Model file for the job. Use its own axes, mm. Face numbers are marked on the shaded views. Coordinates: 2 decimals unless noted, no trailing zeros.
from build123d import *

# Parameters (mm, degrees)
SKETCH_2_R          = 45
CUT_EXTRUDE_1_DEPTH = 15
CUT_EXTRUDE_2_DEPTH = 27
SKETCH_4_W          = 1.65
SKETCH_4_H          = 14.7


with BuildPart() as part:
    # Sketch 1 → Revolve 1 (revolve)
    with BuildSketch(Plane(origin=(0, 0, 0), x_dir=(0, 0, -1), z_dir=(1, 0, 0)), mode=Mode.PRIVATE) as revolve_1_sk:
        Polygon((-15, 19.5), (-15, 6.3), (-14.7, 6), (-0.3, 6), (0, 6.3), (0, 19.5), (-0.803847577, 22.5), (-14.196152423, 22.5), align=None)
    revolve(revolve_1_sk.sketch.rotate(Axis((0, 0, 0), (0, 0, 1)), 270), axis=Axis((0, 0, 0), (0, 0, 1)))

    # Sketch 2 → Cut-Extrude 1 (cut)
    with BuildSketch(Plane.XY):
        Circle(SKETCH_2_R)
        Polygon((-22.5, 0), (-19.377388093, -2.183307284), (-21.935878024, -5.006721014), (-18.405724941, -6.440441708), (-20.271799528, -9.76238413), (-16.511121885, -10.374625492), (-17.591208356, -14.028520542), (-13.788582233, -13.788582233), (-14.028520542, -17.591208356), (-10.374625492, -16.511121885), (-9.76238413, -20.271799528), (-6.440441708, -18.405724941), (-5.006721014, -21.935878024), (-2.183307284, -19.377388093), (0, -22.5), (2.183307284, -19.377388093), (5.006721014, -21.935878024), (6.440441708, -18.405724941), (9.76238413, -20.271799528), (10.374625492, -16.511121885), (14.028520542, -17.591208356), (13.788582233, -13.788582233), (17.591208356, -14.028520542), (16.511121885, -10.374625492), (20.271799528, -9.76238413), (18.405724941, -6.440441708), (21.935878024, -5.006721014), (19.377388093, -2.183307284), (22.5, 0), (19.377388093, 2.183307284), (21.935878024, 5.006721014), (18.405724941, 6.440441708), (20.271799528, 9.76238413), (16.511121885, 10.374625492), (17.591208356, 14.028520542), (13.788582233, 13.788582233), (14.028520542, 17.591208356), (10.374625492, 16.511121885), (9.76238413, 20.271799528), (6.440441708, 18.405724941), (5.006721014, 21.935878024), (2.183307284, 19.377388093), (0, 22.5), (-2.183307284, 19.377388093), (-5.006721014, 21.935878024), (-6.440441708, 18.405724941), (-9.76238413, 20.271799528), (-10.374625492, 16.511121885), (-14.028520542, 17.591208356), (-13.788582233, 13.788582233), (-17.591208356, 14.028520542), (-16.511121885, 10.374625492), (-20.271799528, 9.76238413), (-18.405724941, 6.440441708), (-21.935878024, 5.006721014), (-19.377388093, 2.183307284), align=None, mode=Mode.SUBTRACT)
    extrude(amount=CUT_EXTRUDE_1_DEPTH, mode=Mode.SUBTRACT)

    # Sketch 3 → Cut-Extrude 2 (cut)
    with BuildSketch(Plane.XY):
        with BuildLine():
            Line((-2, 0), (2, 0))
            Line((2, 0), (2, 7.6))
            ThreePointArc((2, 7.6), (1.941421356, 7.741421356), (1.8, 7.8))
            Line((1.8, 7.8), (-1.8, 7.8))
            ThreePointArc((-1.8, 7.8), (-1.941421356, 7.741421356), (-2, 7.6))
            Line((-2, 7.6), (-2, 0))
        make_face()
    extrude(amount=CUT_EXTRUDE_2_DEPTH, mode=Mode.SUBTRACT)

    # Sketch 4 → Hole Wizard M4 _1 (revolve, cut)
    with BuildSketch(Plane(origin=(0, 7.8, 7.5), x_dir=(0, 0, -1), z_dir=(1, 0, 0))):
        with Locations((0.825, 7.35)):
            Rectangle(SKETCH_4_W, SKETCH_4_H)
    revolve(axis=Axis((0, 1.45, 7.5), (0, 1, 0)), mode=Mode.SUBTRACT)


solid = part.part
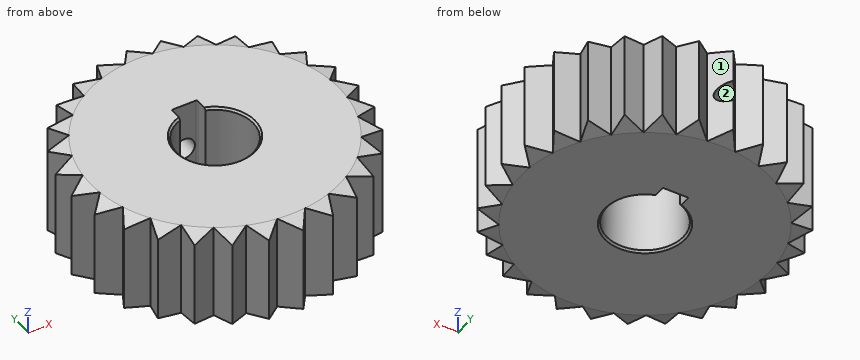
Q1. Drill centre lines: line 1 (Z direction, x = 0, y = 13); line 2 (X direction, y = -19.5, z = 13); line 3 (Y direction, x = 21.5, z = 13). Where is each one in solid material? Low to high.
Answers:
line 1: z = 0 to 5.85, 9.15 to 15
line 2: x = -9.89 to -8.39, -6 to -2.32, -2.1 to 2.1, 2.32 to 6, 8.39 to 9.89
line 3: y = -5.18 to -4.53, -0.7 to 0.7, 4.53 to 5.18
Q2. Flat gauge pins, fed straight in: P1, Ø2, axis at y = -18, z = 11.5, coming from the -X side; P2, Ø8, axis at y = 14.5, z = 5.5, coming from the +X side; P3, Ø1.6, axis at y = 7, z = 4, coming from the -X side. Where does each tip first touch, or does it go through?
Answers:
P1: stops at x = -14.03
P2: stops at x = 17.59
P3: stops at x = -19.17
Q3. Mould opens along Z. For the marked faces 1 and 2 say: +Z half, -Z half, draft (parallel to the pull), parting line (faces both ways), or undercut.
Answers:
face 1: draft
face 2: undercut
